from build123d import *

# Parameters (mm, degrees)
SKETCH1_R           = 2.25
BOSS_EXTRUDE1_DEPTH = 8
SKETCH1_3_R         = 1.375
BOSS_EXTRUDE2_DEPTH = 1
SKETCH5_R           = 1.25
BOSS_EXTRUDE3_DEPTH = 1
SKETCH6_R           = 2
BOSS_EXTRUDE4_DEPTH = 1
SKETCH12_R          = 1.4
CUT_EXTRUDE1_DEPTH  = 7.5


with BuildPart() as part:
    # Sketch1 → Boss-Extrude1 (new body)
    with BuildSketch(Plane(origin=(0, 0, 0), x_dir=(1, 0, 0), z_dir=(0, 1, 0))):
        with Locations((-0.522013312, 0.511138034)):
            Circle(SKETCH1_R)
    extrude(amount=BOSS_EXTRUDE1_DEPTH)

    # Sketch1<3> → Boss-Extrude2 (add)
    with BuildSketch(Plane(origin=(0, 0, 0), x_dir=(1, 0, 0), z_dir=(0, 1, 0))):
        with Locations((-0.522013312, 0.511138034)):
            Circle(SKETCH1_3_R)
    extrude(amount=BOSS_EXTRUDE2_DEPTH)

    # Sketch5 → Boss-Extrude3 (add)
    with BuildSketch(Plane.XZ):
        with Locations((-0.522013312, -0.511138034)):
            Circle(SKETCH5_R)
    extrude(amount=BOSS_EXTRUDE3_DEPTH)

    # Sketch6 → Boss-Extrude4 (add)
    with BuildSketch(Plane.XZ.offset(1)):
        with Locations((-0.522013312, -0.511138034)):
            Circle(SKETCH6_R)
    extrude(amount=BOSS_EXTRUDE4_DEPTH)

    # Sketch12 → Cut-Extrude1 (cut)
    with BuildSketch(Plane(origin=(0, 8, 0), x_dir=(1, 0, 0), z_dir=(0, 1, 0))):
        with Locations((-0.522013312, 0.511138034)):
            Circle(SKETCH12_R)
    extrude(amount=-CUT_EXTRUDE1_DEPTH, mode=Mode.SUBTRACT)


solid = part.part
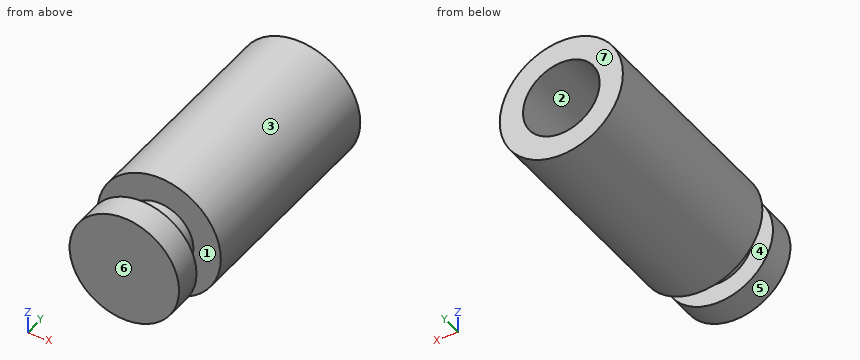
Model file for the job. Use its own axes, mm. Face numbers are marked on the shaded views. A direction names the side the tool comes from. Give positions to 0.01 mm unless a question says otherwise; leave off trailing zeros. Loops run counter-clockwise (first coordinate to the right, second up) from the corner with the lowest first, then second, coordinate; pieces in that order, holes last. Notation, with made-up numbers: (32.25, 45.5) -> (83.25, 45.5) arc R28 ccw to (83.25, 75.5) -> close; hole circle Ø4 at (-8.75, 55). An arc over 180 degrees is marked (long way). Use a Markdown table: item, result. Add a question column.
(1) Slice it at C-C on y = 6.75. List the corners of the cut face in (x, z).
(2) Tool access for the marked faces 1, 2 and 3: list every direction of +Z, -Z, +X, -X, +Y, -Y with a clear straight run to the whole face (end or side of a thin tool).
(3) Mould opens along Y. For the marked faces 4, 5, 6 and 7 say: +Y half, -Y half, draft (parallel to the pull), parting line (faces both ways), or undercut.
(4) Slice it at D-D on y = -0.5. List the corners of the cut face in (x, z), and give its area (3 significant figures).
(5) Wall check: line 1 along Y through (x, z) = (-0.25, 1.4); line 2 along Z through (x, y) = (-0.55, 1); line 3 along Z through (x, y) = (-0.3, 5.25). Give the ranges that are in metal, low to high.
(6) Drop flat-ended pins along their axis: pin 1 Ø1.4 at (x, z) = (-1, -0.5) entering from +Y; pin 2 Ø1 at (x, y) = (-2, 1.5) entering from +Z. Give the stop position or say it passes through.
(7) Slice it at B-B on z = -1.55. List the corners of the cut face in (x, y).
(8) Slice it at A-A on x = -0.4. List the corners of the cut face in (y, z).
Filled sheet:
| question | item | result |
|---|---|---|
| 1 | outline | circle Ø4.5 at (-0.52, -0.51); hole circle Ø2.8 at (-0.52, -0.51) |
| 2 | face 1 | none |
| 2 | face 2 | +Y |
| 2 | face 3 | +Y, -Y |
| 3 | face 4 | undercut |
| 3 | face 5 | draft |
| 3 | face 6 | -Y half |
| 3 | face 7 | +Y half |
| 4 | outline | circle Ø2.5 at (-0.52, -0.51) |
| 4 | area | 4.91 mm2 |
| 5 | line 1 | -2 to -1, 0 to 8 |
| 5 | line 2 | -2.76 to -1.91, 0.89 to 1.74 |
| 5 | line 3 | -2.75 to -1.89, 0.87 to 1.73 |
| 6 | pin 1 | y = 0.5 |
| 6 | pin 2 | z = 1.52 |
| 7 | outline | (-2.52, 0) -> (-1.22, 0) -> (-1.22, -1) -> (-2.23, -1) -> (-2.23, -2) -> (1.19, -2) -> (1.19, -1) -> (0.17, -1) -> (0.17, 0) -> (1.47, 0) -> (1.47, 8) -> (0.42, 8) -> (0.42, 0.5) -> (-1.46, 0.5) -> (-1.46, 8) -> (-2.52, 8) -> close |
| 8 | outline | (-2, -2.51) -> (-1, -2.51) -> (-1, -1.76) -> (0, -1.76) -> (0, -2.76) -> (8, -2.76) -> (8, -1.91) -> (0.5, -1.91) -> (0.5, 0.88) -> (8, 0.88) -> (8, 1.74) -> (0, 1.74) -> (0, 0.73) -> (-1, 0.73) -> (-1, 1.49) -> (-2, 1.49) -> close |
